```python
from build123d import *

# Parameters (mm, degrees)
EXTRUDE_1_DEPTH          = 2.7
EXTRUDE_1_DEPTH_BACK     = 2.7
EXTRUDE_2_DEPTH          = 1
EXTRUDE_2_DEPTH_BACK     = 1
CUT_EXTRUDE_1_DEPTH      = 30.222251796
PATTERN_LINEAR_1_COUNT   = 3
PATTERN_LINEAR_1_PITCH   = 7.5
EXTRUDE_3_DEPTH          = 2
EXTRUDE_3_DEPTH_BACK     = 2
CUT_EXTRUDE_2_DEPTH      = 2
CUT_EXTRUDE_2_DEPTH_BACK = 2
FILLET_1_R               = 0.1
FILLET_4_R               = 0.2
FILLET_5_R               = 0.2
FILLET_8_R               = 0.2


with BuildPart() as part:
    # 草图1 → 凸台-拉伸1 (new, two sides: drawn at the far end of the back side and taken through both)
    with BuildSketch(Plane.XY.offset(-EXTRUDE_1_DEPTH_BACK)):
        Polygon((0, 0), (7.5, 0), (7.5, 2), (-7.5, 2), (-7.5, 0), align=None)
    extrude(amount=EXTRUDE_1_DEPTH + EXTRUDE_1_DEPTH_BACK)

    # 草图2 → 凸台-拉伸2 (add, two sides: drawn at the far end of the back side and taken through both)
    with BuildSketch(Plane.XY.offset(-EXTRUDE_2_DEPTH_BACK)):
        with BuildLine():
            Line((-7.5, 2), (-5.474663278, 23.027315834))
            ThreePointArc((-5.474663278, 23.027315834), (0, 28), (5.474663278, 23.027315834))
            Line((5.474663278, 23.027315834), (7.5, 2))
            Line((7.5, 2), (-7.5, 2))
        make_face()
    extrude(amount=EXTRUDE_2_DEPTH + EXTRUDE_2_DEPTH_BACK)

    # 草图3 → 切除-拉伸1 (cut, through all)
    with BuildSketch(Plane.XY.offset(1)):
        with BuildLine():
            Line((3.5, 6), (3.5, 9))
            Line((3.5, 9), (1.322875656, 9))
            ThreePointArc((1.322875656, 9), (0, 9.5), (-1.322875656, 9))
            Line((-1.322875656, 9), (-3.5, 9))
            Line((-3.5, 9), (-3.5, 6))
            Line((-3.5, 6), (-1.322875656, 6))
            ThreePointArc((-1.322875656, 6), (0, 5.5), (1.322875656, 6))
            Line((1.322875656, 6), (3.5, 6))
        make_face()
    cut_extrude_1 = extrude(amount=-CUT_EXTRUDE_1_DEPTH, mode=Mode.SUBTRACT)

    # 阵列(线性)1: 切除-拉伸1 ×3
    with Locations(*[(0, i * PATTERN_LINEAR_1_PITCH, 0) for i in range(1, PATTERN_LINEAR_1_COUNT)]):
        add(cut_extrude_1, mode=Mode.SUBTRACT)

    # 草图4 → 凸台-拉伸3 (add, two sides: drawn at the far end of the back side and taken through both)
    with BuildSketch(Plane.XY.offset(-EXTRUDE_3_DEPTH_BACK)):
        with BuildLine():
            Line((1.5, 0), (-1.5, 0))
            Line((-1.5, 0), (-1.5, -0.677124344))
            ThreePointArc((-1.5, -0.677124344), (-1.780042303, -1.088161527), (-1.95, -1.555590279))
            Line((-1.95, -1.555590279), (-1.95, -2.5))
            Line((-1.95, -2.5), (1.95, -2.5))
            Line((1.95, -2.5), (1.95, -1.555590279))
            ThreePointArc((1.95, -1.555590279), (1.780042303, -1.088161527), (1.5, -0.677124344))
            Line((1.5, -0.677124344), (1.5, 0))
        make_face()
    extrude(amount=EXTRUDE_3_DEPTH + EXTRUDE_3_DEPTH_BACK)

    # 草图5 → 切除-拉伸2 (cut, two sides: drawn at the far end of the back side and taken through both)
    with BuildSketch(Plane(origin=(0, 0, 0), x_dir=(0, 0, -1), z_dir=(1, 0, 0)).offset(-CUT_EXTRUDE_2_DEPTH_BACK)):
        with BuildLine():
            Line((1.5, 0), (1.5, -0.677124344))
            ThreePointArc((1.5, -0.677124344), (1.780042303, -1.088161527), (1.95, -1.555590279))
            Line((1.95, -1.555590279), (1.95, -2.5))
            Line((1.95, -2.5), (2, -2.5))
            Line((2, -2.5), (2, 0))
            Line((2, 0), (1.5, 0))
        make_face()
        with BuildLine():
            Line((-2, 0), (-1.5, 0))
            Line((-1.5, 0), (-1.5, -0.677124344))
            ThreePointArc((-1.5, -0.677124344), (-1.780042303, -1.088161527), (-1.95, -1.555590279))
            Line((-1.95, -1.555590279), (-1.95, -2.5))
            Line((-1.95, -2.5), (-2, -2.5))
            Line((-2, -2.5), (-2, 0))
        make_face()
    extrude(amount=CUT_EXTRUDE_2_DEPTH + CUT_EXTRUDE_2_DEPTH_BACK, mode=Mode.SUBTRACT)

    # 圆角1
    fillet_1_edges = [part.edges().sort_by_distance(p)[0] for p in [
        (-1.95, -2.5, 0),
        (1.95, -2.5, 0),
        (0, -2.5, -1.95),
        (0, -2.5, 1.95),
    ]]
    fillet(fillet_1_edges, radius=FILLET_1_R)

    # 圆角4
    fillet_4_edges = [part.edges().sort_by_distance(p)[0] for p in [
        (-7.5, 1, 2.7),
        (0, 2, 2.7),
        (7.5, 1, 2.7),
        (0, 0, 2.7),
        (7.5, 1, -2.7),
        (0, 2, -2.7),
        (-7.5, 1, -2.7),
        (0, 0, -2.7),
    ]]
    fillet(fillet_4_edges, radius=FILLET_4_R)

    # 圆角5
    # the kernel refuses this fillet: 0.2 mm, written as the material it takes off along each edge
    with BuildSketch(Plane(origin=(7.3, 0.2, 2.5), x_dir=(1, 0, 0), z_dir=(0, -1, 0))) as fillet_5_piece_1_section:
        Polygon((0, 0), (FILLET_5_R, 0), (FILLET_5_R, FILLET_5_R), (0, FILLET_5_R), align=None)
    fillet_5_piece_1 = extrude(amount=FILLET_5_R, mode=Mode.PRIVATE)
    fillet_5_piece_1 = fillet_5_piece_1 - Plane(origin=(7.3, 0.2, 2.5), x_dir=(-0.7071067811865475, 0, -0.7071067811865475), z_dir=(0, -1, 0)) * Sphere(FILLET_5_R, mode=Mode.PRIVATE)
    add(fillet_5_piece_1, mode=Mode.SUBTRACT)
    with BuildSketch(Plane(origin=(-7.3, 0.2, 2.5), x_dir=(-1, 0, 0), z_dir=(0, -1, 0))) as fillet_5_piece_2_section:
        Polygon((0, 0), (FILLET_5_R, 0), (FILLET_5_R, -FILLET_5_R), (0, -FILLET_5_R), align=None)
    fillet_5_piece_2 = extrude(amount=FILLET_5_R, mode=Mode.PRIVATE)
    fillet_5_piece_2 = fillet_5_piece_2 - Plane(origin=(-7.3, 0.2, 2.5), x_dir=(0.7071067811865475, 1.2560739669470211e-15, -0.7071067811865475), z_dir=(0, -1, 0)) * Sphere(FILLET_5_R, mode=Mode.PRIVATE)
    add(fillet_5_piece_2, mode=Mode.SUBTRACT)
    with BuildSketch(Plane(origin=(-7.3, 0.2, -2.5), x_dir=(-1, 0, 0), z_dir=(0, -1, 0))) as fillet_5_piece_3_section:
        Polygon((0, 0), (FILLET_5_R, 0), (FILLET_5_R, FILLET_5_R), (0, FILLET_5_R), align=None)
    fillet_5_piece_3 = extrude(amount=FILLET_5_R, mode=Mode.PRIVATE)
    fillet_5_piece_3 = fillet_5_piece_3 - Plane(origin=(-7.3, 0.2, -2.5), x_dir=(0.7071067811865475, 1.2560739669470211e-15, 0.7071067811865475), z_dir=(0, -1, 0)) * Sphere(FILLET_5_R, mode=Mode.PRIVATE)
    add(fillet_5_piece_3, mode=Mode.SUBTRACT)
    with BuildSketch(Plane(origin=(7.3, 0.2, -2.5), x_dir=(1, 0, 0), z_dir=(0, -1, 0))) as fillet_5_piece_4_section:
        Polygon((0, 0), (FILLET_5_R, 0), (FILLET_5_R, -FILLET_5_R), (0, -FILLET_5_R), align=None)
    fillet_5_piece_4 = extrude(amount=FILLET_5_R, mode=Mode.PRIVATE)
    fillet_5_piece_4 = fillet_5_piece_4 - Plane(origin=(7.3, 0.2, -2.5), x_dir=(-0.7071067811865475, 0, 0.7071067811865475), z_dir=(0, -1, 0)) * Sphere(FILLET_5_R, mode=Mode.PRIVATE)
    add(fillet_5_piece_4, mode=Mode.SUBTRACT)
    with BuildSketch(Plane(origin=(-7.5, 0, 2.5), x_dir=(1, 0, 0), z_dir=(0, 0, -1)), Plane(origin=(7.5, 0, -2.5), x_dir=(-1, 0, 0), z_dir=(0, 0, 1))) as fillet_5_piece_5:
        with BuildLine():
            CenterArc((FILLET_5_R, -FILLET_5_R), FILLET_5_R, 90, 90)
            Line((0, -FILLET_5_R), (0, 0))
            Line((0, 0), (FILLET_5_R, 0))
        make_face()
    extrude(amount=5, mode=Mode.SUBTRACT)

    # 圆角8
    # the kernel refuses this fillet: 0.2 mm, written as the material it takes off along each edge
    with BuildSketch(Plane(origin=(-7.547937803, 1.502303338, 1), x_dir=(0, 0, -1), z_dir=(0.09587560610090687, 0.9953933233424785, 0))) as fillet_8_piece_1_section:
        with BuildLine():
            CenterArc((FILLET_8_R, -FILLET_8_R), FILLET_8_R, 90, 90)
            Line((0, -FILLET_8_R), (0, 0))
            Line((0, 0), (FILLET_8_R, 0))
        make_face()
    fillet_8_piece_1 = extrude(amount=21.624630174, mode=Mode.PRIVATE)
    fillet_8_piece_1 = split(fillet_8_piece_1, bisect_by=Plane(origin=(-6.442060612, 2, 0.954715968), z_dir=(0, 1, 0)), keep=Keep.TOP, mode=Mode.PRIVATE)
    add(fillet_8_piece_1, mode=Mode.SUBTRACT)
    with BuildSketch(Plane(origin=(5.474663278, 23.027315834, -1), x_dir=(0, 0, 1), z_dir=(0.09587560610090687, -0.9953933233424785, 0))) as fillet_8_piece_2_section:
        with BuildLine():
            CenterArc((FILLET_8_R, FILLET_8_R), FILLET_8_R, 180, 90)
            Line((0, FILLET_8_R), (0, 0))
            Line((0, 0), (FILLET_8_R, 0))
        make_face()
    fillet_8_piece_2 = extrude(amount=21.624630174, mode=Mode.PRIVATE)
    fillet_8_piece_2 = split(fillet_8_piece_2, bisect_by=Plane(origin=(6.442060612, 2, -0.954715968), z_dir=(0, 1, 0)), keep=Keep.TOP, mode=Mode.PRIVATE)
    add(fillet_8_piece_2, mode=Mode.SUBTRACT)
    with BuildSketch(Plane(origin=(0, 22.5, -1), x_dir=(-0.9953933233424784, 0.09587560610090734, 0), z_dir=(-0.09587560610090734, -0.9953933233424784, 0))) as fillet_8_piece_3:
        with BuildLine():
            CenterArc((5.5 - FILLET_8_R, -FILLET_8_R), FILLET_8_R, 0, 90)
            Line((5.5, -FILLET_8_R), (5.5, 0))
            Line((5.5, 0), (5.5 - FILLET_8_R, 0))
        make_face()
    revolve(axis=Axis((0, 22.5, -1), (0, 0, -1)), revolution_arc=168.996563204, mode=Mode.SUBTRACT)
    with BuildSketch(Plane(origin=(-7.547937803, 1.502303338, -1), x_dir=(0, 0, 1), z_dir=(0.09587560610090687, 0.9953933233424785, 0))) as fillet_8_piece_4_section:
        with BuildLine():
            CenterArc((FILLET_8_R, FILLET_8_R), FILLET_8_R, 180, 90)
            Line((0, FILLET_8_R), (0, 0))
            Line((0, 0), (FILLET_8_R, 0))
        make_face()
    fillet_8_piece_4 = extrude(amount=21.624630174, mode=Mode.PRIVATE)
    fillet_8_piece_4 = split(fillet_8_piece_4, bisect_by=Plane(origin=(-6.442060612, 2, -0.954715968), z_dir=(0, 1, 0)), keep=Keep.TOP, mode=Mode.PRIVATE)
    add(fillet_8_piece_4, mode=Mode.SUBTRACT)
    with BuildSketch(Plane(origin=(0, 22.5, 1), x_dir=(-0.9953933233424784, 0.09587560610090734, 0), z_dir=(-0.09587560610090734, -0.9953933233424784, 0))) as fillet_8_piece_5:
        with BuildLine():
            CenterArc((5.5 - FILLET_8_R, FILLET_8_R), FILLET_8_R, 270, 90)
            Line((5.5 - FILLET_8_R, 0), (5.5, 0))
            Line((5.5, 0), (5.5, FILLET_8_R))
        make_face()
    revolve(axis=Axis((0, 22.5, 1), (0, 0, -1)), revolution_arc=168.996563204, mode=Mode.SUBTRACT)
    with BuildSketch(Plane(origin=(5.474663278, 23.027315834, 1), x_dir=(0, 0, -1), z_dir=(0.09587560610090687, -0.9953933233424785, 0))) as fillet_8_piece_6_section:
        with BuildLine():
            CenterArc((FILLET_8_R, -FILLET_8_R), FILLET_8_R, 90, 90)
            Line((0, -FILLET_8_R), (0, 0))
            Line((0, 0), (FILLET_8_R, 0))
        make_face()
    fillet_8_piece_6 = extrude(amount=21.624630174, mode=Mode.PRIVATE)
    fillet_8_piece_6 = split(fillet_8_piece_6, bisect_by=Plane(origin=(6.442060612, 2, 0.954715968), z_dir=(0, 1, 0)), keep=Keep.TOP, mode=Mode.PRIVATE)
    add(fillet_8_piece_6, mode=Mode.SUBTRACT)


solid = part.part
```
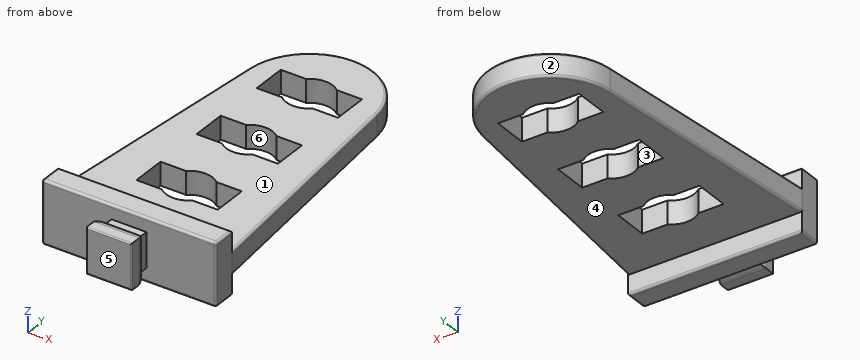
Verification items for the finished model (mm, model axes). Face numbers are marked on the shaded views. A direction names the side the tool comes from. Round coordinates to 2 decimals unless told otherwise and drop trailing zeros. Answer as a JSON object with one key per item and string values. Group by question number.
Q1. Go/stop test with flat-tipped pins: pin 1 Ø0.5 at (x, y) = (-0.5, -0.5) entering from +Z; pin 2 Ø1 at (x, z) = (3, -0.5) entering from +Y; pin 3 Ø1.6 at (x, z) = (-2, -0.5) entering from +Y; pin 4 Ø0.6 at (x, z) = (2, 0) entering from -Y. Record where each tip stops, or that it passes through.
Q2. Section check A-A, the plane z = -0.5. Give the number of separate pieces and of enclosed holes in the cut face, plus the area to 3 significant figures.
Q3. Tool access check on the marked faces 4, 5 and 6. Record the directions out of +Z, -Z, +X, -X, +Y, -Y that give a thin tool (end or side, any length) a straight path to the whole face; none if there is none.
Q4. Mould release check, pull along X, two halves, no side actions. Record for the marked faces 1, 2 and 3: released by +X, released by -X, zero draft, split by the parting line, or undercut.
Q5. Thickness scan on line 1 (Y direction, x = -3, z = -0.4); line 2 (Y direction, x = -0.5, z = 2.45); line 3 (Y direction, x = -1, z = 1.1). Record the ranges inside material, lowest first.
Found:
{
 "1": {"pin 1": "stops at z = 1.56", "pin 2": "stops at y = 27.4", "pin 3": "stops at y = 27.87", "pin 4": "stops at y = -2.5"},
 "2": {"separate pieces": "1", "enclosed holes": "3", "area": "285 mm^2"},
 "3": {"face 4": "-Z, +X, -X, +Y", "face 5": "+Z, -Z, +X, -X, -Y", "face 6": "+Z, -Z"},
 "4": {"face 1": "zero draft", "face 2": "split by the parting line", "face 3": "undercut"},
 "5": {"line 1": "y = 0 to 6, 9 to 13.5, 16.5 to 21, 24 to 27.11", "line 2": "y = 0 to 2", "line 3": "y = -2.5 to 2"}
}
